Autodesk Inventor part; units mm, degrees
ref_plane "YZ Plane" through (0, 0, 0) normal (1, 0, 0) x (0, 1, 0)
ref_plane "XZ Plane" through (0, 0, 0) normal (0, 1, 0) x (-1, 0, 0)
ref_plane "XY Plane" through (0, 0, 0) normal (0, 0, 1) x (1, 0, 0)
sketch "Sketch1" plane through (0, 0, 0) normal (0, 0, 1) x (1, 0, 0)
  line L0 (0, 0) -> (4.445, 0)
  line L1 (4.445, 0) -> (4.445, 20.32)
  line L2 (4.445, 20.32) -> (0, 20.32)
  line L3 (0, 20.32) -> (0, 0)
  dimension "d0" = 4.445
  dimension "d1" = 20.32
extrude "Extrusion1" add sketch "Sketch1" along normal blind 19.05
chamfer "Chamfer1" distance 16.51 angle 45 1 edges at (2.2225, 20.32, 19.05)
sketch "Sketch2" plane through (0, 0, 0) normal (0, -1, 0) x (1, 0, 0)
  line L0 (0, 19.05) -> (4.445, 19.05)
  line L1 (0, 0) -> (4.445, 0)
  line L2 (0, 3.429) -> (4.445, 3.429)
  line L3 (4.445, 3.429) -> (4.445, 7.239)
  line L4 (4.445, 7.239) -> (0, 7.239)
  line L5 (0, 7.239) -> (0, 3.429)
  line L6 (4.445, 0) -> (4.445, 19.05)
  line L7 (0, 11.811) -> (4.445, 11.811)
  line L8 (4.445, 11.811) -> (4.445, 15.621)
  line L9 (4.445, 15.621) -> (0, 15.621)
  line L10 (0, 15.621) -> (0, 11.811)
  dimension "d7" = 19.05
  dimension "d8" = 3.81
  dimension "d9" = 3.81
  dimension "d10" = 4.445
  dimension "d11" = 4.445
  dimension "d12" = 3.429
  dimension "d13" = 3.429
  dimension "d16" = 8.382
extrude "Extrusion2" add sketch "Sketch2" along normal blind 6.35
properties part number "MonsterHolderSupport1"
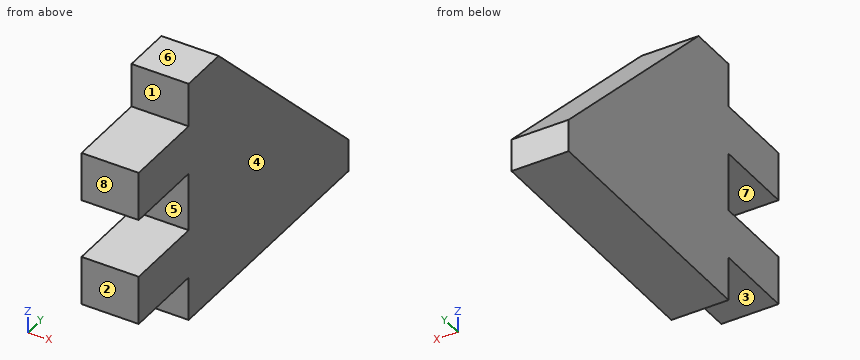
For this review, take the finished solid that the model builds, in its own axes (mm). Face numbers are marked on the shaded views. A direction names the side the tool comes from. Coordinates: 2 decimals unless noted, no trailing zeros. Loops run counter-clockwise (first coordinate to the right, second up) from the corner with the lowest first, then second, coordinate; pieces in that order, holes last. Notation, with made-up numbers: (-39, -35) - (17, -35) arc R21 ccw to (17, -19) - close; hole circle Ø4 at (10, 19). An arc over 180 degrees is marked (long way). Use a Markdown table: item, result. Add a question column.
Item 1: Tool access review of the marked faces 1, 2, 3, 4 and 5: name each direction out of +Z, -Z, +X, -X, +Y, -Y from which nothing blocks a thin tool from reaching the whole face with its end or side.
Item 2: We need section D-D (z = 12.75). Give the boundary of the cut face in (x, y) (3 decimals).
Item 3: Insertion check: pin 1 Ø1.3 at (x, y) = (3, -4.5) entering from +Z; pin 2 Ø1.3 at (x, z) = (2, 9.5) entering from -Y. Each pin has a flat end and moves straight along its axis. Give the tip position at first contact, or say it passes through.
Item 4: For line 1 (Z direction, x = 4, y = -2.25); line 2 (Z direction, x = 3.75, y = 11.5); line 3 (Y direction, x = 2.9, z = 1), list the stretches that pass through material, from the lowest coordinate up.
Item 5: Mouldability with a two-part tool opening along Z and no side actions: class the marked faces 6, 7 and 8 as pulls with the +Z half, pulls with the -Z half, needs draft (parallel to the pull), parting line crosses it, or undercut.
Item 6: We need section C-C (y = 13.75). Give the boundary of the cut face in (x, z) (3 decimals).
Item 7: We need section B-B (x = 1.1). Give the boundary of the cut face in (y, z).
Item 8: We need section A-A (y = -1). Give the boundary of the cut face in (x, z) (3 decimals), and give its area (3 significant figures).
Results list:
| question | item | result |
|---|---|---|
| 1 | face 1 | +Z, +X, -X, -Y |
| 1 | face 2 | +Z, -Z, +X, -X, -Y |
| 1 | face 3 | -Z, +X, -X, -Y |
| 1 | face 4 | +Z, -Z, +X, +Y, -Y |
| 1 | face 5 | +X, -X, -Y |
| 2 | outline | (0, -6.35) - (4.445, -6.35) - (4.445, 10.11) - (0, 10.11) - close |
| 3 | pin 1 | stops at z = 15.62 |
| 3 | pin 2 | stops at y = 0 |
| 4 | line 1 | z = 3.43 to 7.24, 11.81 to 15.62 |
| 4 | line 2 | z = 0 to 11.36 |
| 4 | line 3 | y = 0 to 20.32 |
| 5 | face 6 | pulls with the +Z half |
| 5 | face 7 | undercut |
| 5 | face 8 | needs draft |
| 6 | outline | (0, 0) - (4.445, 0) - (4.445, 9.11) - (0, 9.11) - close |
| 7 | outline | (-6.35, 3.43) - (0, 3.43) - (0, 0) - (20.32, 0) - (20.32, 2.54) - (3.81, 19.05) - (0, 19.05) - (0, 15.62) - (-6.35, 15.62) - (-6.35, 11.81) - (0, 11.81) - (0, 7.24) - (-6.35, 7.24) - close |
| 8 | outline | (0, 3.429) - (4.445, 3.429) - (4.445, 7.239) - (0, 7.239) - close; (0, 11.811) - (4.445, 11.811) - (4.445, 15.621) - (0, 15.621) - close |
| 8 | area | 33.9 mm^2 |
